Check sheet for the modelled part. Datum: model origin and axes. Units: mm. Face numbers are marked on the shaded views. A direction names the side the tool comes from. Coordinates: 2 decimals unless noted, no trailing zeros. Loops run counter-clockwise (first coordinate to the right, second up) from the corner with the lowest first, then second, coordinate; pieces in that order, holes last. Notation, with made-up numbers: (-39.75, 5.5) -> (-15.75, 5.5) arc R21 cw to (-15.75, 16.5) -> close; hole circle Ø8 at (63.25, 41.5). An arc over 180 degrees is marked (long way). Use one line per item in the form item = value.
from build123d import *

# Parameters (mm, degrees)
F0_W     = 81.045844
F0_H     = 87.006435
F1_DEPTH = 129.564196
F2_W     = 51.355398
F2_H     = 51.861688
F3_DEPTH = 421.159267


with BuildPart() as f1:
    # F0 (on Right) → F1 (new body)
    with BuildSketch(Plane.YZ):
        with Locations((40.522922, 43.503217)):
            Rectangle(F0_W, F0_H)
    extrude(amount=F1_DEPTH)

    # F2 (on face) → F3 (join)
    with BuildSketch(Plane.YZ.offset(129.564196)):
        with Locations((40.588942, 42.482689)):
            Rectangle(F2_W, F2_H)
    extrude(amount=-F3_DEPTH)


solid = f1.part
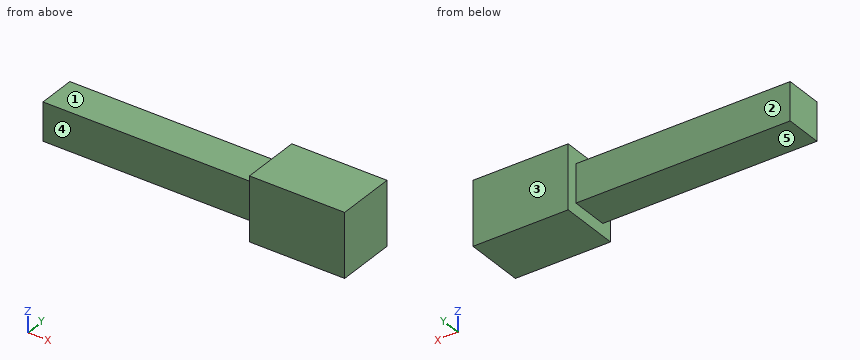
(1) Section check C-C, the plane x = -18. Record the boundary of the cut face in (y, z).
Established:
outline = (14.91, 16.55) -> (66.27, 16.55) -> (66.27, 68.41) -> (14.91, 68.41) -> close
(2) Tool access check on the marked faces 1, 2, 3, 4 and 5. Record the directions out of +Z, -Z, +X, -X, +Y, -Y that give a thin tool (end or side, any length) a straight path to the whole face; none if there is none.
Established:
face_1 = +Z, -X, +Y, -Y
face_2 = +Z, -Z, -X, +Y
face_3 = +Z, -Z, +X, -X, +Y
face_4 = +Z, -Z, -X, -Y
face_5 = -Z, -X, +Y, -Y
(3) Section check D-D, the plane z = 72.5. Record the boundary of the cut face in (x, y).
Established:
outline = (0, 0) -> (129.56, 0) -> (129.56, 81.05) -> (0, 81.05) -> close
(4) Section check A-A, the plane z = 51. Record the boundary of the cut face in (x, y).
Established:
outline = (-291.6, 14.91) -> (0, 14.91) -> (0, 0) -> (129.56, 0) -> (129.56, 81.05) -> (0, 81.05) -> (0, 66.27) -> (-291.6, 66.27) -> close
(5) Go/stop test with flat-tipped pins: P1, Ø2, axis at x = -176, y = 26, coming from the -Z side; P2, Ø15.5, axis at x = -129, z = 52.5, coming from the +Y side; P3, Ø1.5, axis at x = -247, z = 46.5, coming from the -Y side. Record where each tip stops, or that it passes through.
Established:
P1 = 16.55
P2 = 66.27
P3 = 14.91
(6) Section check B-B, the plane y = 31. Record the boundary of the cut face in (x, z), plus the area to 3 significant figures.
Established:
outline = (-291.6, 16.55) -> (0, 16.55) -> (0, 0) -> (129.56, 0) -> (129.56, 87.01) -> (0, 87.01) -> (0, 68.41) -> (-291.6, 68.41) -> close
area = 26,400 mm²
(7) Scan lines: line 1 along Z through (x, y) = (-253, 22.5); line 2 along Y through (x, z) = (-2.5, 22); line 3 along X through (y, z) = (21, 75). Record each from-to range of solid material in increasing order.
Established:
line_1 = 16.55 to 68.41
line_2 = 14.91 to 66.27
line_3 = 0 to 129.56
